from build123d import *

# Parameters (mm, degrees)
ESQUISSE1_W                                       = 50
ESQUISSE1_H                                       = 50
ESQUISSE1_R                                       = 14.5
BOSS_EXTRU_1_DEPTH                                = 10
ESQUISSE2_R                                       = 21.3
BOSS_EXTRU_2_DEPTH                                = 100
CHAMBRAGE_POUR_VIS_SIX_PANS_CREUX_M41_D           = 4.5
CHAMBRAGE_POUR_VIS_SIX_PANS_CREUX_M41_CBORE_D     = 8
CHAMBRAGE_POUR_VIS_SIX_PANS_CREUX_M41_CBORE_DEPTH = 4.4
CHAMBRAGE_POUR_VIS_SIX_PANS_CREUX_M42_D           = 4.8
CHAMBRAGE_POUR_VIS_SIX_PANS_CREUX_M42_CBORE_D     = 8
CHAMBRAGE_POUR_VIS_SIX_PANS_CREUX_M42_CBORE_DEPTH = 4.4
CONG_1_R                                          = 4


with BuildPart() as part:
    # Esquisse1 → Boss.-Extru.1 (new body)
    with BuildSketch(Plane(origin=(0, 0, 0), x_dir=(1, 0, 0), z_dir=(0, 1, 0))):
        with Locations((25, 25)):
            Rectangle(ESQUISSE1_W, ESQUISSE1_H)
        with Locations((25, 25)):
            Circle(ESQUISSE1_R, mode=Mode.SUBTRACT)
    extrude(amount=BOSS_EXTRU_1_DEPTH)

    # Esquisse2 → Boss.-Extru.2 (add)
    with BuildSketch(Plane(origin=(0, 10, 0), x_dir=(1, 0, 0), z_dir=(0, 1, 0))):
        with BuildLine():
            Line((40, 44), (40, 46))
            ThreePointArc((40, 46), (38.828427125, 48.828427125), (36, 50))
            Line((36, 50), (14, 50))
            ThreePointArc((14, 50), (11.171572875, 48.828427125), (10, 46))
            Line((10, 46), (10, 44))
            ThreePointArc((10, 44), (8.828427125, 41.171572875), (6, 40))
            Line((6, 40), (4, 40))
            ThreePointArc((4, 40), (1.171572875, 38.828427125), (0, 36))
            Line((0, 36), (0, 14))
            ThreePointArc((0, 14), (1.171572875, 11.171572875), (4, 10))
            Line((4, 10), (6, 10))
            ThreePointArc((6, 10), (8.828427125, 8.828427125), (10, 6))
            Line((10, 6), (10, 4))
            ThreePointArc((10, 4), (11.171572875, 1.171572875), (14, 0))
            Line((14, 0), (36, 0))
            ThreePointArc((36, 0), (38.828427125, 1.171572875), (40, 4))
            Line((40, 4), (40, 6))
            ThreePointArc((40, 6), (41.171572875, 8.828427125), (44, 10))
            Line((44, 10), (46, 10))
            ThreePointArc((46, 10), (48.828427125, 11.171572875), (50, 14))
            Line((50, 14), (50, 36))
            ThreePointArc((50, 36), (48.828427125, 38.828427125), (46, 40))
            Line((46, 40), (44, 40))
            ThreePointArc((44, 40), (41.171572875, 41.171572875), (40, 44))
        make_face()
        with Locations((25, 25)):
            Circle(ESQUISSE2_R, mode=Mode.SUBTRACT)
    extrude(amount=BOSS_EXTRU_2_DEPTH)

    # Chambrage pour vis à six pans creux M41 (through all)
    with Locations(Plane(origin=(5, 10, -45), x_dir=(0, 0, 1), z_dir=(0, 1, 0))):
        with Locations((0, 0), (0, 40), (40, 40), (40, 0)):
            CounterBoreHole(CHAMBRAGE_POUR_VIS_SIX_PANS_CREUX_M41_D / 2, CHAMBRAGE_POUR_VIS_SIX_PANS_CREUX_M41_CBORE_D / 2, CHAMBRAGE_POUR_VIS_SIX_PANS_CREUX_M41_CBORE_DEPTH)

    # Chambrage pour vis à six pans creux M42 (through all)
    with Locations(Plane(origin=(25, 0, -7.5), x_dir=(0, 0, -1), z_dir=(0, -1, 0))):
        with Locations((0, 0), (17.5, 17.5), (35, 0), (17.5, -17.5)):
            CounterBoreHole(CHAMBRAGE_POUR_VIS_SIX_PANS_CREUX_M42_D / 2, CHAMBRAGE_POUR_VIS_SIX_PANS_CREUX_M42_CBORE_D / 2, CHAMBRAGE_POUR_VIS_SIX_PANS_CREUX_M42_CBORE_DEPTH)

    # Congé1
    cong_1_edges = [part.edges().sort_by_distance(p)[0] for p in [
        (0, 5, -50),
        (50, 5, -50),
        (50, 5, 0),
        (0, 5, 0),
    ]]
    fillet(cong_1_edges, radius=CONG_1_R)


solid = part.part
The listing builds one solid part. Answer for the finished solid, in the listing's coordinates (mm). A direction names the side the tool comes from. Round coordinates to 2 decimals unless told otherwise and drop trailing zeros. Write each loop counter-clockwise with the first axis right and the second up, starting at its lowest first coordinate (ties: lowest second). Pieces come first, ordered by that corner, then holes. Notation, with made-up numbers: M 73,-6 L 117,-6 A6 cw 117,-1 Z; hole C 79,-2 d11. An arc over 180 degrees is marked long. Write each question's results on one line, items separated by ' | '. Start each with the question number.
Item 1: For a pull along Z with two mould halves and no side action, classify faces 4 (the face through (25, 54, -50)), 5 (the face through (20, 10, -11)), 6 (the face through (7, 10, -9)) as pulls with the +Z half, pulls with the -Z half, needs draft (parallel to the pull), parting line crosses it, or undercut.
Item 2: A cutting plane is placed at B-B on y = 8. State how many separate pieces and enclosed holes the cut face has, and give its area (3 significant figures).
Item 3: Straight lines are drawn through the part: L1, parallel to X at y = 8, z = -25; L2, parallel to X at y = 7.9, z = -45; L3, parallel to X at y = 2.4, z = -42.5. For each, find the intervals that lie inside material, in ascending order. Write a range as [from, to].
Item 4: A cutting plane is placed at C-C on z = -25. Write down the section's boundary in (x, y), and give its area (3 significant figures).
Item 5: Flat-ended cylindrical pins translate along their axes: pin 1 Ø0.6 at (x, y) = (45.5, 36.5) entering from -Z; pin 2 Ø2.5 at (x, z) = (46, -45.5) entering from +Y; pin 3 Ø7 at (x, z) = (42.5, -25) entering from +Y; pin 4 Ø4 at (x, z) = (5, -5) entering from -Y. Find the tip coordinate at first contact, or state that the pin passes through.
Item 6: For faces 1 (the face through (26.8, 4.4, -44.4)), 2 (the face through (11.203, 59.3, -48.859)), 3 (the face through (38.797, 59.3, -1.141)), determine the directions among +Z, -Z, +X, -X, +Y, -Y from which every point of the face is accessible in a straight line to the end or side of a thin tool.
Item 7: A cutting plane is placed at A-A on x = 25. Write down the section's boundary in (y, z).
Item 8: A cutting plane is placed at D-D on z = -16. Write down the section's boundary in (x, y).
Check sheet entries:
1) face 4: pulls with the -Z half | face 5: undercut | face 6: needs draft
2) separate pieces: 1 | enclosed holes: 9 | area: 1,550 mm²
3) L1: [0, 5.1], [9.9, 10.5], [39.5, 40.1], [44.9, 50] | L2: [0, 1], [9, 41], [49, 50] | L3: [0, 21], [29, 50]
4) outline: M 0,0 L 3.5,0 L 3.5,4.4 L 5.1,4.4 L 5.1,10 L 3.7,10 L 3.7,110 L 0,110 Z; M 9.9,4.4 L 10.5,4.4 L 10.5,10 L 9.9,10 Z; M 39.5,4.4 L 40.1,4.4 L 40.1,10 L 39.5,10 Z; M 44.9,4.4 L 46.5,4.4 L 46.5,0 L 50,0 L 50,110 L 46.3,110 L 46.3,10 L 44.9,10 Z | area: 835 mm²
5) pin 1: z = -40 | pin 2: y = 5.6 | pin 3: y = 10 | pin 4: through
6) face 1: -Y | face 2: -Z, -X, +Y | face 3: +Z, +X, +Y
7) outline: M 0,-50 L 110,-50 L 110,-46.3 L 10,-46.3 L 10,-44.9 L 4.4,-44.9 L 4.4,-46.5 L 0,-46.5 Z; M 0,-3.5 L 4.4,-3.5 L 4.4,-5.1 L 10,-5.1 L 10,-3.7 L 110,-3.7 L 110,0 L 0,0 Z; M 4.4,-40.1 L 10,-40.1 L 10,-39.5 L 4.4,-39.5 Z; M 4.4,-10.5 L 10,-10.5 L 10,-9.9 L 4.4,-9.9 Z
8) outline: M 0,0 L 13.63,0 L 13.63,10 L 5.69,10 L 5.69,110 L 0,110 Z; M 36.37,0 L 50,0 L 50,110 L 44.31,110 L 44.31,10 L 36.37,10 Z
